```python
from build123d import *

# Parameters (mm, degrees)
SKETCH_1_W               = 71.4
SKETCH_1_H               = 59
EXTRUDE_1_DEPTH          = 3.5
CUT_EXTRUDE_4_DEPTH      = 8.5
CUT_EXTRUDE_4_DEPTH_BACK = 15
SKETCH_2_R               = 1.55
SKETCH_5_W               = 26.11
SKETCH_5_H               = 45.8
EXTRUDE_2_DEPTH          = 10.15
SKETCH_6_W               = 20
SKETCH_6_H               = 39.55
CUT_EXTRUDE_5_DEPTH      = 10.15
SKETCH_9_W               = 5.05
SKETCH_9_H               = 10.15
CUT_EXTRUDE_6_DEPTH      = 10
SKETCH_12_W              = 0.1
SKETCH_12_H              = 3.125
CUT_EXTRUDE_7_DEPTH      = 10


with BuildPart() as part:
    # 草圖1 → 填料-伸長1 (new body)
    with BuildSketch(Plane(origin=(0, 0, 0), x_dir=(1, 0, 0), z_dir=(0, 1, 0))):
        Rectangle(SKETCH_1_W, SKETCH_1_H)
    extrude(amount=-EXTRUDE_1_DEPTH)

    # 草圖2 → 除料-伸長4 (cut, two sides: drawn at the far end of the back side and taken through both)
    with BuildSketch(Plane(origin=(0, 0, 0), x_dir=(1, 0, 0), z_dir=(0, 1, 0)).offset(-CUT_EXTRUDE_4_DEPTH_BACK)):
        with Locations(Location((20.453418067, -24.130543915, 0), (0, 0, 270))):
            Circle(SKETCH_2_R)
        with Locations(Location((-30.223577589, 18.9, 0), (0, 0, 270))):
            Circle(SKETCH_2_R)
        with Locations(Location((-30.223577589, -8.577967438, 0), (0, 0, 270))):
            Circle(SKETCH_2_R)
        with Locations(Location((21.85, 24.05, 0), (0, 0, 270))):
            Circle(SKETCH_2_R)
    extrude(amount=CUT_EXTRUDE_4_DEPTH + CUT_EXTRUDE_4_DEPTH_BACK, mode=Mode.SUBTRACT)

    # 草圖5 → 填料-伸長2 (add)
    with BuildSketch(Plane(origin=(0, -3.5, 0), x_dir=(-1, 0, 0), z_dir=(0, -1, 0))):
        Rectangle(SKETCH_5_W, SKETCH_5_H)
    extrude(amount=EXTRUDE_2_DEPTH)

    # 草圖6 → 除料-伸長5 (cut)
    with BuildSketch(Plane.XZ.offset(13.65)):
        Rectangle(SKETCH_6_W, SKETCH_6_H)
    extrude(amount=-CUT_EXTRUDE_5_DEPTH, mode=Mode.SUBTRACT)

    # 草圖9 → 除料-伸長6 (cut)
    with BuildSketch(Plane.XY.offset(22.9)):
        with Locations((0, -8.575)):
            Rectangle(SKETCH_9_W, SKETCH_9_H)
    extrude(amount=-CUT_EXTRUDE_6_DEPTH, mode=Mode.SUBTRACT)

    # 草圖12 → 除料-伸長7 (cut)
    with BuildSketch(Plane.XZ.offset(13.65)):
        with Locations((-2.575, 21.3375)):
            Rectangle(SKETCH_12_W, SKETCH_12_H)
        with Locations((2.575, 21.3375)):
            Rectangle(SKETCH_12_W, SKETCH_12_H)
    extrude(amount=-CUT_EXTRUDE_7_DEPTH, mode=Mode.SUBTRACT)


solid = part.part
```
The listing builds one solid part. Answer for the finished solid, in the listing's coordinates (mm). A direction names the side the tool comes from. Coordinates: 2 decimals unless noted, no trailing zeros. Write each loop counter-clockwise with the first axis right and the second up, starting at its lowest first coordinate (ties: lowest second). Pieces come first, ordered by that corner, then holes. Notation, with made-up numbers: (89.5, 87.5) -> (148.5, 87.5) arc R28 cw to (148.5, 111.5) -> close; hole circle Ø11 at (-2, -5). An arc over 180 degrees is marked (long way). Write each question's results on one line, items separated by ' | '. Start each with the question number.
1) For a pull along Z with two mould halves and no side action, classify faces 1 (the flat face through (8, -9, 22.9)), 2 (the cylindrical face through (20.92, -1.77, 25.61)), 3 (the flat face through (-35.7, -2, 0)) as +Z half, -Z half, draft (parallel to the pull), parting line (faces both ways), or undercut.
2) A cutting plane is placed at A-A (z = -24.05). Determine the outline of the cut face in (x, y), then the cut area to 3 significant figures.
3) Flat-ended cylindrical pins translate along their axes: pin 1 Ø3 at (x, z) = (14.5, -9.5) entering from +Y; pin 2 Ø3 at (x, y) = (3.5, -11) entering from +Z; pin 3 Ø8 at (x, y) = (14.5, -10.5) entering from -Z; pin 4 Ø5 at (y, z) = (-8.5, -5.5) entering from -X (3 decimals). Find the tip coordinate at first contact, or state that the pin passes through.
4) A cutting plane is placed at B-B (x = 6.5). Determine the outline of the cut face in (y, z) (3 decimals).
5) A tool of negligible diameter and unlimited length cuts with its end or side. For faces 4 (the flat face through (6, -9, 19.775)), 5 (the flat face through (-8, -9, 22.9)), 6 (the flat face through (-13.055, -9, 0)), 7 (the flat face through (0, -9, -22.9)), from which of +Z, -Z, +X, -X, +Y, -Y can it reach the whole face along a straight path? Write none if from no direction.
6) A cutting plane is placed at C-C (y = -11.25). Determine the outline of the cut face in (x, z) (3 decimals).
7) Straight lines are drawn through the part: probe 1 along Z at (x, y) = (21.85, -1.05); probe 2 along X at (y, z) = (-7.5, -10.5) (3 decimals); probe 3 along X at (y, z) = (-1.45, -24.05). For each, find the intervals that lie inside material, in ascending order.
Values follow:
1) face 1: +Z half | face 2: undercut | face 3: draft
2) outline: (-35.7, -3.5) -> (20.3, -3.5) -> (20.3, 0) -> (-35.7, 0) -> close; (23.4, -3.5) -> (35.7, -3.5) -> (35.7, 0) -> (23.4, 0) -> close | area: 239 mm²
3) pin 1: y = 0 | pin 2: z = 22.9 | pin 3: z = -22.9 | pin 4: x = -13.055
4) outline: (-13.65, -22.9) -> (-3.5, -22.9) -> (-3.5, -29.5) -> (0, -29.5) -> (0, 29.5) -> (-3.5, 29.5) -> (-3.5, 22.9) -> (-13.65, 22.9) -> (-13.65, 19.775) -> (-3.5, 19.775) -> (-3.5, -19.775) -> (-13.65, -19.775) -> close
5) face 4: -Y | face 5: +Z, +X, -X, -Y | face 6: +Z, -Z, -X, -Y | face 7: -Z, +X, -X, -Y
6) outline: (-13.055, -22.9) -> (13.055, -22.9) -> (13.055, 22.9) -> (2.625, 22.9) -> (2.625, 19.775) -> (10, 19.775) -> (10, -19.775) -> (-10, -19.775) -> (-10, 19.775) -> (-2.625, 19.775) -> (-2.625, 22.9) -> (-13.055, 22.9) -> close
7) probe 1: -29.5 to -25.6, -22.5 to 23.46, 24.8 to 29.5 | probe 2: -13.055 to -10, 10 to 13.055 | probe 3: -35.7 to 20.3, 23.4 to 35.7
